Can you work these out from the model? Positions are in its coordinate system, mm. Face numbers are marked on the shaded views. Round coordinates to 2 decimals unless told otherwise and drop trailing zeros. Order: outer loops, then holes, each group sorted by start corner. A loop starts at its lowest first (then second) coordinate and runs counter-clockwise, first axis right, second up. Notation, with made-up numbers: M 66.25,58.25 L 85.25,58.25 A11 cw 85.25,71.25 Z; hole C -11.5,-18 d5. An arc over 180 degrees is marked long. Answer as a JSON object with one key per item and string values. Group by question number.
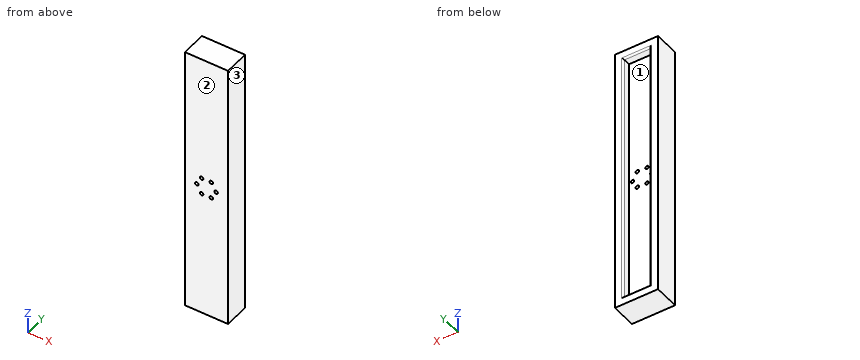
Autodesk Inventor part; units mm, degrees
ref_plane "YZ Plane" through (0, 0, 0) normal (1, 0, 0) x (0, 1, 0)
ref_plane "XZ Plane" through (0, 0, 0) normal (0, 1, 0) x (-1, 0, 0)
ref_plane "XY Plane" through (0, 0, 0) normal (0, 0, 1) x (1, 0, 0)
sketch "Sketch1" plane through (0, 0, 0) normal (0, 1, 0) x (-1, 0, 0)
  line L0 (-15.7, -152.5) -> (15.7, -152.5)
  line L1 (15.7, -152.5) -> (15.7, 152.5)
  line L2 (15.7, 152.5) -> (-15.7, 152.5)
  line L3 (-15.7, 152.5) -> (-15.7, -152.5)
  line L4 (-15.7, -152.5) -> (15.7, 152.5) construction
  line L5 (15.7, -152.5) -> (-15.7, 152.5) construction
  line L6 (25.7, 162.5) -> (25.7, -162.5)
  line L7 (25.7, -162.5) -> (-25.7, -162.5)
  line L8 (-25.7, -162.5) -> (-25.7, 162.5)
  line L9 (-25.7, 162.5) -> (25.7, 162.5)
  point P0 (0, 0)
  dimension "d0" = 31.4
  dimension "d1" = 305
  dimension "d2" = 10
extrude "Extrusion1" add sketch "Sketch1" along normal blind 10
sketch "Sketch2" plane through (0, 0, 0) normal (0, -1, 0) x (1, 0, 0)
  line L0 (25.7, 162.5) -> (25.7, -162.5)
  line L1 (-25.7, 162.5) -> (25.7, 162.5)
  line L2 (-25.7, -162.5) -> (-25.7, 162.5)
  line L3 (25.7, -162.5) -> (-25.7, -162.5)
  line L4 (-15.7, 152.5) -> (-15.7, -152.5)
  line L5 (15.7, 152.5) -> (-15.7, 152.5)
  line L6 (15.7, -152.5) -> (15.7, 152.5)
  line L7 (-15.7, -152.5) -> (15.7, -152.5)
  point P0 (0, 0)
extrude "Extrusion2" add sketch "Sketch2" along normal blind 20 contours L0 L3 L2 L1 | L5 L6 L7 L4
sketch "Sketch4" plane through (0, -20, 0) normal (0, -1, 0) x (1, 0, 0)
  point P0 (0, 0)
  point P1 (11.5, 0)
  dimension "d14" = 11.5
hole "Hole2" at (11.5, -20, 0) direction (0, 1, 0) diameter 4.134 end through all
pattern_circular "Circular Pattern1" count 6 over 360 about axis through (0, -10, 0) along (0, 1, 0) of "Hole2"
fillet "Fillet1" radius 2 4 edges at (-15.7, 10, 0) (0, 10, -152.5) (15.7, 10, 0) (0, 10, 152.5)
properties part number "enclosure_btm"
1) If we section it at A-A on z = 57.5: Write out the boundary of the cut face in (x, y), plus the area to 3 significant figures.
2) For pin 1 (25 mm diameter, centred on x = -1.5, z = -27, fed in from +Y); pin 2 (3.5 mm diameter, centred on x = -5.75, z = 9.96, fed in from -Y), each with a flat end and sliding along its axis, tell me the tip position at first contact or that it passes through.
3) We'd pull the mould along X, two halves only. Please class the marked faces 1, 2 and 3: +X half, -X half, draft (parallel to the pull), parting line (faces both ways), or undercut.
4) I need wall thicknesses on line 1 along Z through (x, y) = (-5.5, -16.75); line 2 along X through (y, z) = (3.5, 125.5); line 3 along Z through (x, y) = (10.5, 3.75). Which ranges of each line are inside material? Lowest first, please.
Findings:
{
 "1": {"outline": "M -25.7,-20 L 25.7,-20 L 25.7,10 L 17.7,10 A2 ccw 15.7,8 L 15.7,0 L -15.7,0 L -15.7,8 A2 ccw -17.7,10 L -25.7,10 Z", "area": "1,230 mm^2"},
 "2": {"pin 1": "stops at y = 0", "pin 2": "passes through"},
 "3": {"face 1": "undercut", "face 2": "draft", "face 3": "+X half"},
 "4": {"line 1": "z = -162.5 to -12.01, -7.91 to 7.91, 12.01 to 162.5", "line 2": "x = -25.7 to -15.7, 15.7 to 25.7", "line 3": "z = -162.5 to -152.5, 152.5 to 162.5"}
}
